Build history of the part. All positions in model axes, mm. Face numbers are marked on the shaded views. Round coordinates to 2 decimals unless told otherwise and drop trailing zeros. Order: outer loops, then holes, each group sorted by start corner. A loop starts at its lowest first (then second) coordinate and runs counter-clockwise, first axis right, second up. Notation, with made-up numbers: (65.5, 71.25) -> (119.5, 71.25) arc R11 ccw to (119.5, 79.25) -> close; hole circle Ø9 at (45, 17.25). An arc over 180 degrees is marked (long way). Answer as CSV lines item,"result". Start each with the question number.
```python
from build123d import *

# Parameters (mm, degrees)
BOSS_EXTRUDE1_DEPTH = 1.5
FILLET1_R           = 2
SKETCH2_R           = 1.95
CUT_EXTRUDE1_DEPTH  = 10


with BuildPart() as part:
    # Sketch1 → Boss-Extrude1 (new body)
    with BuildSketch(Plane(origin=(0, 0, 0), x_dir=(0, 0, -1), z_dir=(1, 0, 0))):
        Polygon((130.053191489, -78.292553191), (230.053191489, -78.292553191), (230.053191489, -140.292553191), (-269.946808511, -140.292553191), (-269.946808511, -78.292553191), (100.053191489, -78.292553191), (100.053191489, -100.292553191), (130.053191489, -100.292553191), align=None)
    extrude(amount=BOSS_EXTRUDE1_DEPTH)

    # Fillet1
    fillet1_edges = [part.edges().sort_by_distance(p)[0] for p in [
        (0.75, -78.292553191, 269.946808511),
        (0.75, -78.292553191, -100.053191489),
        (0.75, -100.292553191, -100.053191489),
        (0.75, -100.292553191, -130.053191489),
        (0.75, -78.292553191, -130.053191489),
        (0.75, -78.292553191, -230.053191489),
        (0.75, -140.292553191, -230.053191489),
        (0.75, -140.292553191, 269.946808511),
    ]]
    fillet(fillet1_edges, radius=FILLET1_R)

    # Sketch2 → Cut-Extrude1 (cut)
    with BuildSketch(Plane.ZY):
        with Locations((-150.053191489, -110.292553191)):
            Circle(SKETCH2_R)
        with Locations((-150.053191489, -130.292553191)):
            Circle(SKETCH2_R)
        with Locations((189.946808511, -110.292553191)):
            Circle(SKETCH2_R)
        with Locations((189.946808511, -130.292553191)):
            Circle(SKETCH2_R)
    extrude(amount=-CUT_EXTRUDE1_DEPTH, mode=Mode.SUBTRACT)


solid = part.part
```
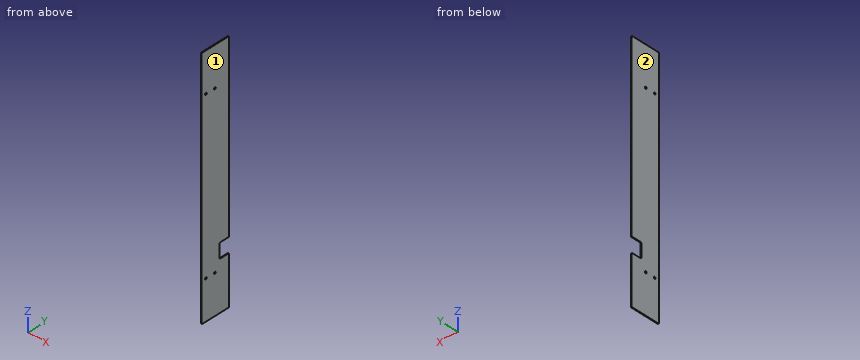
Q1. Probe L1, parallel to Z at x = 0.7, y = -84; L2, parallel to Y at x = 1.1, z = 190; L3, parallel to Z at x = 0.6, y = -99. List the from-to ranges inside material, lowest first.
Q2. Flat gauge pin, fed straight in: pin 1 Ø0.8 at (x, z) = (1, -108.5) entering from +Y. Where does the tip first touch, or does it go through?
Q3. Slice it at A-A, the plane y = -87. Write the cut outline in (x, z), plus the area to 3 significant figures.
Q4. Two-plate mould, pull along X, no slides. Class the marked faces 1 and 2: +X half, -X half, draft (parallel to the pull), parting line (faces both ways), or undercut.
Q5. Slice it at B-B, the plane x = 0.85. Write the cut outline in (y, z), plus the area to 3 significant figures.
Solutions:
1,L1,"z = -230.05 to -130.05, -100.05 to 269.95"
1,L2,"y = -140.29 to -132.24, -128.34 to -112.24, -108.34 to -78.29"
1,L3,"z = -230.05 to -129.92, -100.18 to 269.95"
2,pin 1,"stops at y = -100.29"
3,outline,"(0, -230.05) -> (1.5, -230.05) -> (1.5, -130.05) -> (0, -130.05) -> close; (0, -100.05) -> (1.5, -100.05) -> (1.5, 269.95) -> (0, 269.95) -> close"
3,area,"705 mm2"
4,face 1,"+X half"
4,face 2,"-X half"
5,outline,"(-140.29, -228.05) arc R2 ccw to (-138.29, -230.05) -> (-80.29, -230.05) arc R2 ccw to (-78.29, -228.05) -> (-78.29, -132.05) arc R2 ccw to (-80.29, -130.05) -> (-98.29, -130.05) arc R2 cw to (-100.29, -128.05) -> (-100.29, -102.05) arc R2 cw to (-98.29, -100.05) -> (-80.29, -100.05) arc R2 ccw to (-78.29, -98.05) -> (-78.29, 267.95) arc R2 ccw to (-80.29, 269.95) -> (-138.29, 269.95) arc R2 ccw to (-140.29, 267.95) -> close; hole circle Ø3.9 at (-130.29, -150.05); hole circle Ø3.9 at (-130.29, 189.95); hole circle Ø3.9 at (-110.29, -150.05); hole circle Ø3.9 at (-110.29, 189.95)"
5,area,"30,300 mm2"
